```python
from build123d import *

# Parameters (mm, degrees)
CROQUIS1_R              = 15
SALIENTE_EXTRUIR1_DEPTH = 2.5
SALIENTE_EXTRUIR2_START = 2.5
CROQUIS1_4_R            = 1.75
SALIENTE_EXTRUIR2_DEPTH = 5
CROQUIS2_R              = 7.9
SALIENTE_EXTRUIR3_DEPTH = 10


with BuildPart() as part:
    # Croquis1 → Saliente-Extruir1 (new body)
    with BuildSketch(Plane(origin=(0, 0, 0), x_dir=(1, 0, 0), z_dir=(0, 1, 0))):
        with Locations(Location((0, 0, 0), (0, 0, 270))):
            Circle(CROQUIS1_R)
    extrude(amount=SALIENTE_EXTRUIR1_DEPTH)

    # Croquis1<4> → Saliente-Extruir2 (add)
    with BuildSketch(Plane(origin=(0, 0, 0), x_dir=(1, 0, 0), z_dir=(0, 1, 0)).offset(SALIENTE_EXTRUIR2_START)):
        with Locations(Location((-12.15, 0, 0), (0, 0, 270))):
            Circle(CROQUIS1_4_R)
        with BuildLine():
            ThreePointArc((-6.146996997, -6.777678653), (9.15, 0), (-6.146996997, 6.777678653))
            ThreePointArc((-6.146996997, 6.777678653), (-4.15, 0), (-6.146996997, -6.777678653))
        make_face()
    extrude(amount=SALIENTE_EXTRUIR2_DEPTH)

    # Croquis2 → Saliente-Extruir3 (add)
    with BuildSketch(Plane.XZ):
        with Locations(Location((0, 0, 0), (0, 0, 90))):
            Circle(CROQUIS2_R)
    extrude(amount=SALIENTE_EXTRUIR3_DEPTH)


solid = part.part
```
The listing builds one solid part. Answer for the finished solid, in the listing's coordinates (mm). A direction names the side the tool comes from. Round coordinates to 2 decimals unless told otherwise and drop trailing zeros. Loops run counter-clockwise (first coordinate to the right, second up) from the corner with the lowest first, then second, coordinate; pieces in that order, holes last.
1) Given P1, Ø3, axis at y = -2, z = 8, coming from the -X side; P2, Ø4, axis at x = 10.5, y = 3, coming from the +Z side; P3, Ø10, axis at y = -0.5, z = 11.5, coming from the -X side, each flat-ended and moving along its own axis, determine where each tip first touches the part or whether it passes through.
Outcome:
P1: stops at x = -4.49
P2: stops at z = 12.32
P3: stops at x = -13.51
2) A cutting plane is placed at C-C on z = 0. Determine the outline of the cut face in (x, y).
Outcome:
outline: (-15, 0) - (-7.9, 0) - (-7.9, -10) - (7.9, -10) - (7.9, 0) - (15, 0) - (15, 2.5) - (9.15, 2.5) - (9.15, 7.5) - (-4.15, 7.5) - (-4.15, 2.5) - (-10.4, 2.5) - (-10.4, 7.5) - (-13.9, 7.5) - (-13.9, 2.5) - (-15, 2.5) - close
3) For a pull along X with two mould halves and no side action, classify faces 1 (the face through (-4.15, 4.96, -0.1)), 2 (the face through (-12, 7.5, 0)), 3 (the face through (9.145, 4.965, 0.296)), 4 (the face through (-13.86, 4.96, -0.38)) as released by +X, released by -X, zero draft, split by the parting line, or undercut.
Outcome:
face 1: undercut
face 2: zero draft
face 3: split by the parting line
face 4: undercut
4) A cutting plane is placed at B-B on y = 4. Determine the outline of the cut face in (x, z), plus the area to 3 significant figures.
Outcome:
outline: circle Ø3.5 at (-12.15, 0); (-6.15, -6.78) arc R9.15 ccw (long way) to (-6.15, 6.78) arc R12.5 cw to start
area: 226 mm2
5) For faces 5 (the face through (1, 7.5, 0)), 6 (the face through (-5.34, -4.93, -5.82)), 7 (the face through (-6, 2.5, 0)), determine the directions among +Z, -Z, +X, -X, +Y, -Y from which every point of the face is accessible in a straight line to the end or side of a thin tool.
Outcome:
face 5: +Z, -Z, +X, -X, +Y
face 6: -Y
face 7: +Y
6) Consider line 1 (Y direction, x = 3.25, z = -7.5); line 2 (Z direction, x = -0.25, y = 4.5); line 3 (Y direction, x = -11.5, z = -7.75). Determine where each line is inside the solid, lowest interval first.
Outcome:
line 1: y = 0 to 7.5
line 2: z = -9.15 to 9.15
line 3: y = 0 to 2.5
7) A cutting plane is placed at D-D on x = -12.15. Determine the outline of the cut face in (y, z).
Outcome:
outline: (0, -8.8) - (2.5, -8.8) - (2.5, -1.75) - (7.5, -1.75) - (7.5, 1.75) - (2.5, 1.75) - (2.5, 8.8) - (0, 8.8) - close
8) A cutting plane is placed at A-A on x = 0. Determine the outline of the cut face in (y, z).
Outcome:
outline: (-10, -7.9) - (0, -7.9) - (0, -15) - (2.5, -15) - (2.5, -9.15) - (7.5, -9.15) - (7.5, 9.15) - (2.5, 9.15) - (2.5, 15) - (0, 15) - (0, 7.9) - (-10, 7.9) - close
